```python
from build123d import *

# Parameters (mm, degrees)
SKETCH1_W           = 85.7504
SKETCH1_H           = 53.975
BOSS_EXTRUDE1_DEPTH = 51.054
SKETCH2_W           = 29.21
SKETCH2_H           = 50.8
CUT_EXTRUDE1_DEPTH  = 114.458991011
SKETCH3_W           = 79.4004
SKETCH3_H           = 50.8
CUT_EXTRUDE2_DEPTH  = 7.747
SKETCH4_W           = 79.4004
SKETCH4_H           = 7.747
CUT_EXTRUDE3_DEPTH  = 50.8
FILLET2_R           = 3.175
FILLET3_R           = 3.175
FILLET4_R           = 3.175
FILLET5_R           = 3.175
FILLET6_R           = 3.175


with BuildPart() as part:
    # Sketch1 → Boss-Extrude1 (new body)
    with BuildSketch(Plane(origin=(0, 0, 0), x_dir=(-1, 0, 0), z_dir=(0, 0, -1))):
        with Locations((-42.8752, 26.9875)):
            Rectangle(SKETCH1_W, SKETCH1_H)
    extrude(amount=-BOSS_EXTRUDE1_DEPTH)

    # Sketch2 → Cut-Extrude1 (cut, through all)
    with BuildSketch(Plane.ZY):
        with Locations((25.527, 25.4)):
            Rectangle(SKETCH2_W, SKETCH2_H)
    extrude(amount=-CUT_EXTRUDE1_DEPTH, mode=Mode.SUBTRACT)

    # Sketch3 → Cut-Extrude2 (cut)
    with BuildSketch(Plane.XY.offset(10.922)):
        with Locations((42.8752, 25.4)):
            Rectangle(SKETCH3_W, SKETCH3_H)
    extrude(amount=-CUT_EXTRUDE2_DEPTH, mode=Mode.SUBTRACT)

    # Sketch4 → Cut-Extrude3 (cut)
    with BuildSketch(Plane.XZ):
        with Locations((42.8752, 44.0055)):
            Rectangle(SKETCH4_W, SKETCH4_H)
    extrude(amount=-CUT_EXTRUDE3_DEPTH, mode=Mode.SUBTRACT)

    # Fillet2
    fillet2_edges = [part.edges().sort_by_distance(p)[0] for p in [
        (3.175, 25.4, 3.175),
    ]]
    fillet(fillet2_edges, radius=FILLET2_R)

    # Fillet3
    fillet3_edges = [part.edges().sort_by_distance(p)[0] for p in [
        (44.4627, 50.8, 3.175),
        (3.175, 50.8, 8.636),
        (4.10493597, 50.8, 4.10493597),
    ]]
    fillet(fillet3_edges, radius=FILLET3_R)

    # Fillet4
    fillet4_edges = [part.edges().sort_by_distance(p)[0] for p in [
        (3.175, 50.8, 10.922),
    ]]
    fillet(fillet4_edges, radius=FILLET4_R)

    # Fillet5
    fillet5_edges = [part.edges().sort_by_distance(p)[0] for p in [
        (82.5754, 23.8125, 3.175),
        (82.5754, 50.8, 8.636),
        (82.5754, 49.87006403, 4.10493597),
    ]]
    fillet(fillet5_edges, radius=FILLET5_R)

    # Fillet6
    fillet6_edges = [part.edges().sort_by_distance(p)[0] for p in [
        (82.5754, 50.8, 10.922),
    ]]
    fillet(fillet6_edges, radius=FILLET6_R)


solid = part.part
```
The listing builds one solid part. Answer for the finished solid, in the listing's coordinates (mm). A direction names the side the tool comes from. Round coordinates to 2 decimals unless told otherwise and drop trailing zeros. Order: outer loops, then holes, each group sorted by start corner. A loop starts at its lowest first (then second) coordinate and runs counter-clockwise, first axis right, second up. Notation, with made-up numbers: (81, 30.5) - (94, 30.5) arc R17 cw to (94, 37.5) - close; hole circle Ø8 at (70.25, 13.25). An arc over 180 degrees is marked (long way). Put each result on its own line as item: value. Start each with the question number.
(1) Find section A-A (y = 5.5). Give the vertices of the cut face in (x, z) (3 decimals).
(2) Find section C-C (z = 5). Give the vertices of the cut face in (x, y) (3 decimals), plus the area to 3 significant figures.
(3) Straight lines are drawn through the part: probe 1 along X at (y, z) = (16, 42) (3 decimals); probe 2 along Z at (x, y) = (51, 11) (3 decimals); probe 3 along Y at (x, z) = (27, 43) (3 decimals). For each, find the intervals that lie inside material, in ascending order. Write a range as from..to.
(4) Determine the mould class of faces 4 (the flat face through (43, 27, 0)), 5 (the flat face through (0, 27, 8)), 6 (the flat face through (82.575, 25, 44)) for opening direction X: released by +X, released by -X, zero draft, split by the parting line, or undercut.
(5) Find section D-D (z = 12.5). Give the vertices of the cut face in (x, y) (3 decimals), plus the area to 3 significant figures.
(6) Given P1, Ø21, axis at x = 57.5, z = 31.5, coming from the -Y side, flat-ended and moving along its own axis, determine where the tip first touches the part or whether it passes through.
(7) For faces 1 (the flat face through (84, 25, 40.132)), 2 (the flat face through (43, 27, 51.054)), 3 (the cylindrical face through (43.387, 49.895, 4.13)), determine the directions among +Z, -Z, +X, -X, +Y, -Y from which every point of the face is accessible in a straight line to the end or side of a thin tool.
(8) Find section B-B (x = 59.5). Give the vertices of the cut face in (y, z) (3 decimals), plus the area to 3 significant figures.
Reply:
1. outline: (0, 0) - (85.75, 0) - (85.75, 10.922) - (82.575, 10.922) - (82.575, 6.35) arc R3.175 cw to (79.4, 3.175) - (6.35, 3.175) arc R3.175 cw to (3.175, 6.35) - (3.175, 10.922) - (0, 10.922) - close; (0, 40.132) - (3.175, 40.132) - (3.175, 47.879) - (82.575, 47.879) - (82.575, 40.132) - (85.75, 40.132) - (85.75, 51.054) - (0, 51.054) - close
2. outline: (0, 0) - (3.476, 0) - (3.476, 47.625) arc R2.874 cw to (6.35, 50.499) - (79.4, 50.499) arc R2.874 cw to (82.274, 47.625) - (82.274, 0) - (85.75, 0) - (85.75, 53.975) - (0, 53.975) - close
2. area: 653 mm^2
3. probe 1: 0..3.175, 82.575..85.75
3. probe 2: 0..3.175, 47.879..51.054
3. probe 3: 50.8..53.975
4. face 4: zero draft
4. face 5: released by -X
4. face 6: undercut
5. outline: (0, 50.369) - (4.753, 50.369) arc R3.175 cw to (6.35, 50.8) - (79.4, 50.8) arc R3.175 cw to (80.997, 50.369) - (85.75, 50.369) - (85.75, 53.975) - (0, 53.975) - close
5. area: 277 mm^2
6. P1: y = 50.8
7. face 1: +X, -X, -Y
7. face 2: +Z, +X, -X, +Y, -Y
7. face 3: -Y
8. outline: (0, 0) - (53.975, 0) - (53.975, 51.054) - (0, 51.054) - (0, 47.879) - (50.8, 47.879) - (50.8, 6.35) arc R3.175 cw to (47.625, 3.175) - (0, 3.175) - close
8. area: 487 mm^2
